```python
from build123d import *

# Parameters (mm, degrees)
F2_R     = 5.5245
F3_DEPTH = 13.462
F4_W     = 2.54
F4_H     = 5.842
F5_DEPTH = 11.176
F6_SIZE  = 0.508
F7_SIZE  = 1.27


with BuildPart() as f1:
    # F0 (on Front) → F1 (revolve)
    with BuildSketch(Plane.XZ):
        Polygon((0, 2.54), (0, 0), (11.684, 0), (12.446, 13.716), (9.902083, 13.716), (9.281194, 2.54), align=None)
    revolve(axis=Axis((0, 0, 1.27), (0, 0, 1)))

    # F2 (on face) → F3 (join)
    with BuildSketch(Plane.XY.offset(2.54)):
        Circle(F2_R)
        with BuildLine():
            ThreePointArc((2.527179, 1.587642), (0, -2.9845), (-2.527179, 1.587642))
            Line((-2.527179, 1.587642), (2.527179, 1.587642))
        make_face(mode=Mode.SUBTRACT)
    extrude(amount=F3_DEPTH)

    # F4 (on face) → F5 (join, through all)
    with BuildSketch(Plane.XY.offset(2.54)):
        with Locations((0, 8.001)):
            Rectangle(F4_W, F4_H)
        Polygon((-10.093729, -4.361148), (-8.823729, -6.560852), (-3.764409, -3.639852), (-5.034409, -1.440148), align=None)
        Polygon((8.823729, -6.560852), (10.093729, -4.361148), (5.034409, -1.440148), (3.764409, -3.639852), align=None)
    extrude(amount=F5_DEPTH)

    # F6
    f6_edges = [f1.edges().sort_by_distance(p)[0] for p in [
        (0, 1.587642, 16.002),
        (0, -2.9845, 16.002),
    ]]
    chamfer(f6_edges, length=F6_SIZE)

    # F7
    f7_edges = [f1.edges().sort_by_distance(p)[0] for p in [
        (-11.684, 0, 0),
    ]]
    chamfer(f7_edges, length=F7_SIZE)


solid = f1.part
```
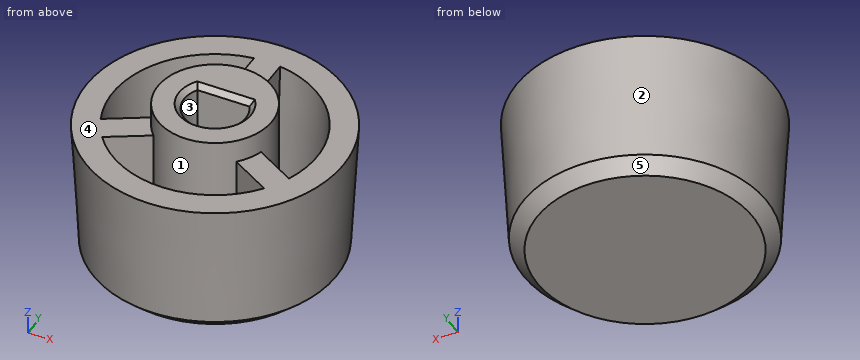
The model under review builds one solid part; all positions refer to its coordinate system, in mm. Face numbers are marked on the shaded views. A direction names the side the tool comes from. Round coordinates to 2 decimals unless told otherwise and drop trailing zeros. Write each loop counter-clockwise with the first axis right and the second up, starting at its lowest first coordinate (ties: lowest second). Pieces come first, ordered by that corner, then holes. Notation, with made-up numbers: (88, 50) - (123, 50) arc R15 cw to (123, 70) - close; hole circle Ø3 at (8.5, 84). An arc over 180 degrees is marked (long way). Use one line per item in the form item = value.
Q1. Insertion check: pin 1 Ø5 at (y, z) = (6.5, 10) entering from +X; pin 2 Ø8 at (x, y) = (8, 1) entering from +Z; pin 3 Ø2 at (x, y) = (-7, 9.5) entering from -Z; pin 4 Ø1.5 at (y, z) = (5.5, 6) entering from +X. Each pin has a flat end and moves straight along its axis. Give the tip position at first contact, or say it passes through.
Answer key:
pin_1 = 11.58
pin_2 = 16
pin_3 = 0.37
pin_4 = 11.04
Q2. Consider section A-A (y = 0). State the section outline as (x, z) points.
Answer key:
outline = (-12.45, 13.72) - (-11.75, 1.27) - (-10.41, 0) - (10.41, 0) - (11.75, 1.27) - (12.45, 13.72) - (9.9, 13.72) - (9.28, 2.54) - (5.52, 2.54) - (5.52, 16) - (3.49, 16) - (2.98, 15.49) - (2.98, 2.54) - (-2.98, 2.54) - (-2.98, 15.49) - (-3.49, 16) - (-5.52, 16) - (-5.52, 2.54) - (-9.28, 2.54) - (-9.9, 13.72) - close
Q3. Draft analysis for pull direction X (two halves, no side actions). For the marked faces 3, 4 and 5, state which applies: +X half, -X half, draft (parallel to the pull), parting line (faces both ways), or undercut.
Answer key:
face_3 = undercut
face_4 = draft
face_5 = parting line
Q4. Consider section B-B (z = 9). State the section outline as (x, y) points.
Answer key:
outline = circle Ø24.37 at (0, 0); hole (-8.91, -3.68) - (-5.29, -1.59) arc R5.52 cw to (-1.27, 5.38) - (-1.27, 9.56) arc R9.64 ccw to start; hole (-7.64, -5.88) arc R9.64 ccw to (7.64, -5.88) - (4.02, -3.79) arc R5.52 cw to (-4.02, -3.79) - close; hole (-2.53, 1.59) arc R2.98 ccw (long way) to (2.53, 1.59) - close; hole (1.27, 5.38) arc R5.52 cw to (5.29, -1.59) - (8.91, -3.68) arc R9.64 ccw to (1.27, 9.56) - close
Q5. Consider section C-C (x = 0). State the section outline as (y, z) points, and give its area (3 significant figures).
Answer key:
outline = (-12.45, 13.72) - (-11.75, 1.27) - (-10.41, 0) - (10.41, 0) - (11.75, 1.27) - (12.45, 13.72) - (5.52, 13.72) - (5.52, 16) - (2.1, 16) - (1.59, 15.49) - (1.59, 2.54) - (-2.98, 2.54) - (-2.98, 15.49) - (-3.49, 16) - (-5.52, 16) - (-5.52, 2.54) - (-9.28, 2.54) - (-9.9, 13.72) - close
area = 247 mm2
Q6. Tool access review of the marked faces 1 and 2: name each direction out of +Z, -Z, +X, -X, +Y, -Y from which nothing blocks a thin tool from reaching the whole face with its end or side.
Answer key:
face_1 = +Z
face_2 = -Z
Q7. Consider section D-D (z = 6). State the section outline as (x, y) points.
Answer key:
outline = circle Ø24.03 at (0, 0); hole (-8.77, -3.59) - (-5.29, -1.59) arc R5.52 cw to (-1.27, 5.38) - (-1.27, 9.39) arc R9.47 ccw to start; hole (-7.5, -5.79) arc R9.47 ccw to (7.5, -5.79) - (4.02, -3.79) arc R5.52 cw to (-4.02, -3.79) - close; hole (-2.53, 1.59) arc R2.98 ccw (long way) to (2.53, 1.59) - close; hole (1.27, 5.38) arc R5.52 cw to (5.29, -1.59) - (8.77, -3.59) arc R9.47 ccw to (1.27, 9.39) - close
Q8. For line 1 (X direction, y = 0, z = 11.75); line 2 (X direction, y = 1, z = 6.5); line 3 (Y direction, x = 0, z = 5.5), list the stretches that pass through material, from the lowest coordinate up. Write a range as [from, to].
Answer key:
line_1 = [-12.34, -9.79], [-5.52, -2.98], [2.98, 5.52], [9.79, 12.34]
line_2 = [-12, -9.45], [-5.43, -2.81], [2.81, 5.43], [9.45, 12]
line_3 = [-11.99, -9.45], [-5.52, -2.98], [1.59, 11.99]
